Autodesk Inventor part; units mm, degrees
ref_plane "YZ Plane" through (0, 0, 0) normal (1, 0, 0) x (0, 1, 0)
ref_plane "XZ Plane" through (0, 0, 0) normal (0, 1, 0) x (-1, 0, 0)
ref_plane "XY Plane" through (0, 0, 0) normal (0, 0, 1) x (1, 0, 0)
sketch "Sketch1" plane through (0, 0, 0) normal (0, 1, 0) x (-1, 0, 0)
  circle A0 centre (0, 0) radius 135
  circle A1 centre (0, 0) radius 110
  dimension "d0" = 270
  dimension "d1" = 220
extrude "Extrusion1" add sketch "Sketch1" along normal mid plane 20
sketch "Sketch3" plane through (0, 10, 0) normal (0, 1, 0) x (1, 0, 0)
  circle A0 centre (0, 0) radius 127.5
  circle A1 centre (127.5, 0) radius 2.5
  circle A2 centre (103.1497, 74.9426) radius 2.5
  circle A3 centre (39.3997, 121.2597) radius 2.5
  circle A4 centre (-39.3997, 121.2597) radius 2.5
  circle A5 centre (-103.1497, 74.9426) radius 2.5
  circle A6 centre (-127.5, 0) radius 2.5
  circle A7 centre (-103.1497, -74.9426) radius 2.5
  circle A8 centre (-39.3997, -121.2597) radius 2.5
  circle A9 centre (39.3997, -121.2597) radius 2.5
  circle A10 centre (103.1497, -74.9426) radius 2.5
  dimension "d7" = 255
  dimension "d8" = 5
  dimension "d11" = 360
hole "Hole1" at (127.5, 10, 0) at (103.1497, 10, 74.9426) at (39.3997, 10, 121.2597) at (-39.3997, 10, 121.2597) at (-103.1497, 10, 74.9426) at (-127.5, 10, 0) at (-103.1497, 10, -74.9426) at (-39.3997, 10, -121.2597) at (39.3997, 10, -121.2597) at (103.1497, 10, -74.9426) direction (0, -1, 0) diameter 5.5 end through all
sketch "Sketch4" plane through (0, 10, 0) normal (0, 1, 0) x (1, 0, 0)
  circle A0 centre (0, 0) radius 110
  circle A1 centre (0, 0) radius 65
  dimension "d21" = 130
extrude "Extrusion3" add sketch "Sketch4" against normal blind 2
sketch "Sketch5" plane through (0, 10, 0) normal (0, 1, 0) x (1, 0, 0)
  line L0 (73.0625, -175) -> (-73.0625, -175)
  line L1 (-73.0625, -175) -> (-73.0625, 175)
  line L2 (-73.0625, 175) -> (73.0625, 175)
  line L3 (73.0625, 175) -> (73.0625, -175)
  line L4 (73.0625, -175) -> (-73.0625, 175) construction
  line L5 (-73.0625, -175) -> (73.0625, 175) construction
  line L6 (73.0625, 0) -> (-74.6125, 0)
  point P0 (0, 0)
  point P1 (-73.0625, 0)
  dimension "d24" = 146.125
  dimension "d25" = 350
extrude "Extrusion4" cut sketch "Sketch5" against normal through all contours L0 L1 L6 L3
properties part number "Cylinder Spacer 25mm"
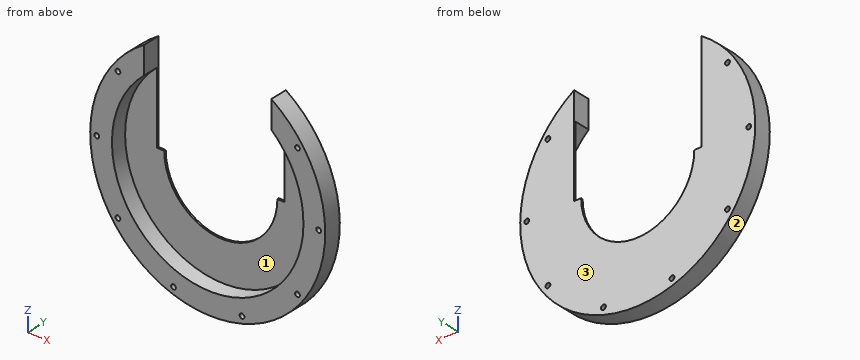
Source: CAD feature listing. Evaluate the final solid. Frame: model axes, mm. Face numbers are marked on the shaded views. Give positions to 0.01 mm unless a question says otherwise; leave off trailing zeros. Order: outer loops, then holes, each group sorted by start corner. A loop starts at its lowest first (then second) coordinate and runs counter-clockwise, first axis right, second up.
(1) Pull-direction query (X, two-part tool) for the marked faces 1, 2 and 3; classes: +X half, -X half, draft (parallel to the pull), parting line (faces both ways), or undercut.
(2) Section query A-A (z = -37). Return the cut outline in (x, y), plus the area to 3 significant figures.
(3) Section query C-C (y = 2.5). State how many separate pieces and enclosed holes the cut face has, plus the area to 3 significant figures.
(4) Section query B-B (x = 0). Return the cut outline in (y, z), plus the area to 3 significant figures.
(5) Contact query for flat-ended pins moving along their axis: P1, Ø3.5, axis at x = 127.5, z = 0, coming from the -Y side; P2, Ø6, axis at y = 3.5, z = 32, coming from the +X side; P3, Ø1.5, axis at x = 77, y = -4.5, coming from the +Z side; P4, Ø0.6, axis at x = 68, y = 9.5, coming from the +Z side. Output: stop coordinate, or through.
(6) Material intervals for line 1 along Z through (x, y) = (-101.5, -4.25); line 2 along X through (y, z) = (-6.75, -74); line 3 along Y through (x, z) = (81.5, -57.5), sorted ascending.
(7) Section query D-D (x = 96). Return the cut outline in (y, z).
Outcome:
1. face 1: undercut
1. face 2: parting line
1. face 3: draft
2. outline: (-129.83, -10) - (-103.59, -10) - (-103.59, 8) - (-53.44, 8) - (-53.44, 10) - (-129.83, 10) - close; (53.44, 8) - (103.59, 8) - (103.59, -10) - (129.83, -10) - (129.83, 10) - (53.44, 10) - close
2. area: 1,250 mm2
3. separate pieces: 1
3. enclosed holes: 8
3. area: 15,100 mm2
4. outline: (-10, -135) - (10, -135) - (10, -65) - (8, -65) - (8, -110) - (-10, -110) - close
4. area: 590 mm2
5. P1: passes through
5. P2: stops at x = 131.85
5. P3: stops at z = 111.4
5. P4: stops at z = 0
6. line 1: z = -89.01 to -77.14, -72.74 to -42.4, 42.4 to 72.74, 77.14 to 89.01
6. line 2: x = -112.91 to -105.73, -100.57 to -81.39, 81.39 to 100.57, 105.73 to 112.91
6. line 3: y = 8 to 10
7. outline: (-10, -94.92) - (10, -94.92) - (10, 94.92) - (-10, 94.92) - (-10, 53.7) - (8, 53.7) - (8, -53.7) - (-10, -53.7) - close
